Source: three-view drawing plus pictorial views. Frame: mm from the lowest corner of the part. A direction names the side the tool comes from. Coordinates: 2 decimals unless noted, no trailing zeros. Write each loop counter-clockwise with the first axis right and the second up, starting at its lowest first coordinate (ties: lowest second). Pieces come first, ordered by that corner, then holes. Notation, with made-up numbers: M 45.5,-17.5 L 91.5,-17.5 A30 cw 91.5,16.5 Z; hole C 75.5,-23 d1. An arc over 180 degrees is marked long. Answer as a JSON object with one key per item and string values. Group by question number.
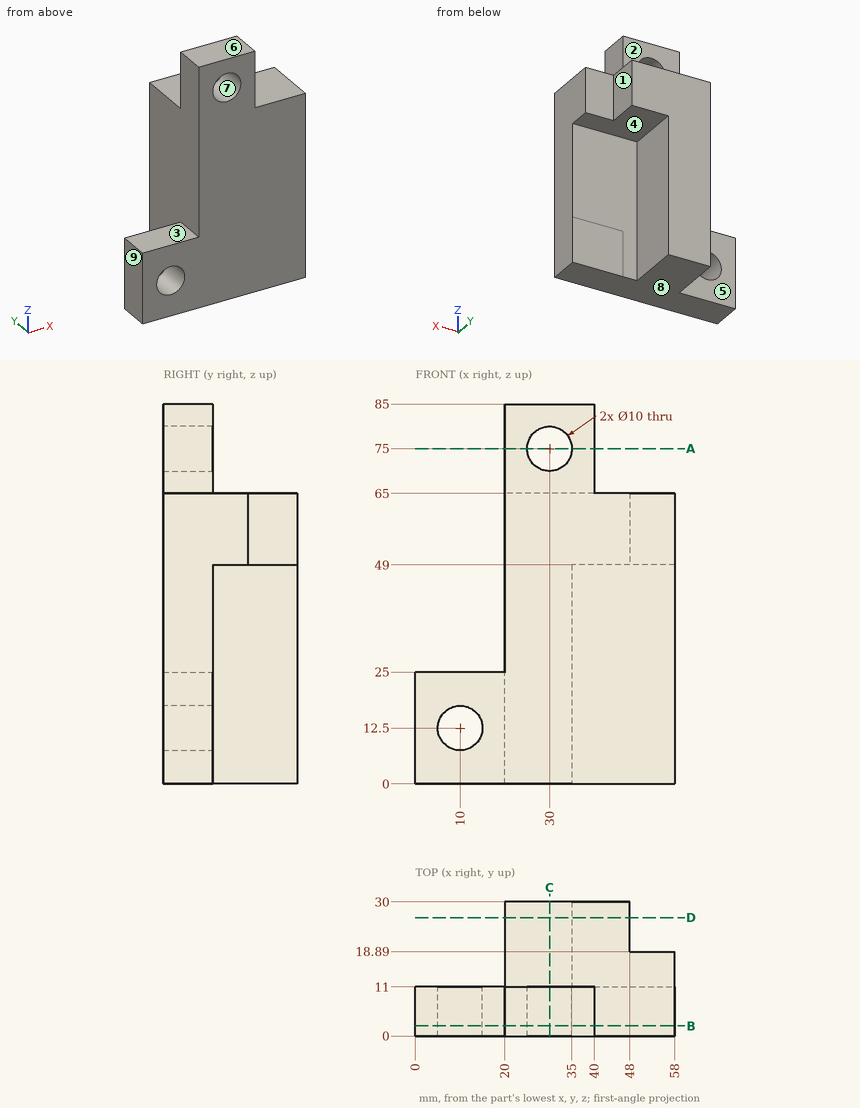
Q1. Section B-B, the plane y = 2.25. Return the cut outline in (x, z).
Q2. Access query for the marked faces 1, 2, 3, 4 and 5. Directions: +Z, -Z, +X, -X, +Y, -Y. A direction counts if a zero-diameter tool reaches every point of the face in a straight line with its end or side. Return the directions, or none.
Q3. Section C-C, the plane x = 30. Return the cut outline in (y, z), and give its area (3 significant figures).
Q4. Draft query along Z for the marked faces 6, 7, 8 and 9. Return one class per face: released by +Z, released by -Z, zero draft, split by the parting line, or undercut.
Q5. Line query: line 1 (Z direction, x = 30, y = 4.75); line 2 (X direction, y = 5.75, z = 75); line 3 (X direction, y = 21.5, z = 61). Output: solid intervals per line, ascending. Write a range as from..to.
Q6. Section A-A, the plane z = 75. Return the cut outline in (x, y).
Q7. Section D-D, the plane y = 26.5. Return the cut outline in (x, z), and give its area (3 significant figures).
Q8. Pin query (flat end, axial travel): pin 1 Ø5.5 at (y, z) = (5.5, 76) entering from +X; pin 2 Ø13 at (x, z) = (45, 5.5) entering from +Y; pin 3 Ø2 at (y, z) = (27, 57) entering from +X. Return the tip coordinate at first contact, or that it passes through.
Filled in:
{
 "1": {"outline": "M 0,0 L 58,0 L 58,65 L 40,65 L 40,85 L 20,85 L 20,25 L 0,25 Z; hole C 10,12.5 d10; hole C 30,75 d10"},
 "2": {"face 1": "+Z, -Z, +X, +Y", "face 2": "+Z, +X, -X, +Y", "face 3": "+Z, -X, +Y, -Y", "face 4": "-Z, +X, +Y", "face 5": "+Z, -Z, -X, +Y"},
 "3": {"outline": "M 0,0 L 30,0 L 30,65 L 11,65 L 11,70 L 0,70 Z; M 0,80 L 11,80 L 11,85 L 0,85 Z", "area": "2,060 mm^2"},
 "4": {"face 6": "released by +Z", "face 7": "undercut", "face 8": "released by -Z", "face 9": "zero draft"},
 "5": {"line 1": "0..70, 80..85", "line 2": "20..25, 35..40", "line 3": "20..48"},
 "6": {"outline": "M 20,0 L 25,0 L 25,11 L 20,11 Z; M 35,0 L 40,0 L 40,11 L 35,11 Z"},
 "7": {"outline": "M 20,0 L 35,0 L 35,49 L 48,49 L 48,65 L 20,65 Z", "area": "1,180 mm^2"},
 "8": {"pin 1": "x = 40", "pin 2": "y = 11", "pin 3": "x = 48"}
}
